Can you work these out from the model? Positions are in its coordinate system, mm. Face numbers are marked on the shaded views. A direction names the side the tool comes from. Round coordinates to 2 decimals unless told otherwise and drop trailing zeros. Order: outer loops, then holes, each group sorted by start corner. A loop starts at its lowest first (then second) coordinate and runs counter-clockwise, first axis right, second up. Notation, with made-up numbers: (-20, -6) -> (7, -6) arc R9 ccw to (7, 4) -> close; hole circle Ø5 at (19.5, -15). An arc over 180 degrees is marked (long way). Use a Markdown table: item, result. Add a question column.
Q1. I'm going to push flat-ended pins straight in: pin 1 Ø2 at (x, z) = (5, 12) entering from +Y; pin 2 Ø3 at (x, z) = (4, 12.5) entering from -Y; pin 3 Ø1.2 at (y, z) = (6, 11) entering from -X. Where does each tip first touch, or does it pass through?
Q2. If we section it at A-A on y = 6: List the corners of the cut face in (x, z) for me, plus the area to 3 significant figures.
Q3. I need wall thicknesses on line 1 along Z through (x, y) = (1, 7); line 2 along X through (y, z) = (5.95, 11). Which ranges of each line are inside material? Lowest first, please. Write a range as [from, to].
Q4. If we section it at D-D on x = 9: List the corners of the cut face in (y, z) for me, plus the area to 3 significant figures.
Q5. If we section it at C-C on z = 12.75: List the corners of the cut face in (x, y) for me.
Q6. For the marked faces 1, 2, 3, 4 and 5, which set-ups out of +Z, -Z, +X, -X, +Y, -Y let a thin tool reach every point of the face, with its end or its side?
Q7. If we section it at B-B on x = 4.25: List the corners of the cut face in (y, z) for me, plus the area to 3 significant figures.
```python
from build123d import *

# Parameters (mm, degrees)
BOX_W              = 10
BOX_H              = 10
BOX_DEPTH          = 10
SKETCH_W           = 4.4
SKETCH_H           = 4.4
PAD_DEPTH          = 4
PAD_FACE4_W        = 10
PAD_FACE4_H        = 10
POCKET_DEPTH       = 2.5
POCKET_FACE5_W     = 10
POCKET_FACE5_H     = 10
POCKET001_DEPTH    = 2.5
SKETCH001_W        = 5
SKETCH001_H        = 10
PAD001_DEPTH       = 10
SKETCH002_W        = 4.4
SKETCH002_H        = 4.4
PAD002_DEPTH       = 4
PAD002_FACE22_W    = 4.4
PAD002_FACE22_H    = 4.4
POCKET002_DEPTH    = 5
POCKET002_FACE16_W = 5
POCKET002_FACE16_H = 10
POCKET003_DEPTH    = 7.5
POCKET003_FACE15_W = 5
POCKET003_FACE15_H = 10
POCKET004_DEPTH    = 2.5
PAD003_DEPTH       = 5


with BuildPart() as part:
    # Box → Box (new body)
    with BuildSketch(Plane.XY):
        with Locations((5, 5)):
            Rectangle(BOX_W, BOX_H)
    extrude(amount=BOX_DEPTH)

    # Sketch (on Face6 of BaseFeature) → Pad (new body)
    with BuildSketch(Plane.XY.offset(10)):
        with Locations((5, 5)):
            Rectangle(SKETCH_W, SKETCH_H)
    extrude(amount=PAD_DEPTH)

    # Pad Face4 → Pocket (cut)
    with BuildSketch(Plane(origin=(5, 10, 5), x_dir=(1, 0, 0), z_dir=(0, 1, 0))):
        Rectangle(PAD_FACE4_W, PAD_FACE4_H)
    extrude(amount=-POCKET_DEPTH, mode=Mode.SUBTRACT)

    # Pocket Face5 → Pocket001 (cut)
    with BuildSketch(Plane(origin=(5, 0, 5), x_dir=(-1, 0, 0), z_dir=(0, -1, 0))):
        Rectangle(POCKET_FACE5_W, POCKET_FACE5_H)
    extrude(amount=-POCKET001_DEPTH, mode=Mode.SUBTRACT)

    # Sketch001 (on Face3 of Pocket001) → Pad001 (join)
    with BuildSketch(Plane(origin=(0, 7.5, 0), x_dir=(-1, 0, 0), z_dir=(0, 1, 0))):
        with Locations((-5, 5)):
            Rectangle(SKETCH001_W, SKETCH001_H)
    extrude(amount=PAD001_DEPTH)

    # Sketch002 (on Face6 of Pad001) → Pad002 (join)
    with BuildSketch(Plane.XY.offset(10)):
        with Locations((5, 12.5)):
            Rectangle(SKETCH002_W, SKETCH002_H)
    extrude(amount=PAD002_DEPTH)

    # Pad002 Face22 → Pocket002 (cut)
    with BuildSketch(Plane(origin=(5, 12.5, 14), x_dir=(0, 1, 0), z_dir=(0, 0, 1))):
        Rectangle(PAD002_FACE22_W, PAD002_FACE22_H)
    extrude(amount=-POCKET002_DEPTH, mode=Mode.SUBTRACT)

    # Pocket002 Face16 → Pocket003 (cut)
    with BuildSketch(Plane(origin=(5, 17.5, 5), x_dir=(1, 0, 0), z_dir=(0, 1, 0))):
        Rectangle(POCKET002_FACE16_W, POCKET002_FACE16_H)
    extrude(amount=-POCKET003_DEPTH, mode=Mode.SUBTRACT)

    # Pocket003 Face15 → Pocket004 (cut)
    with BuildSketch(Plane(origin=(5, 10, 5), x_dir=(1, 0, 0), z_dir=(0, 1, 0))):
        Rectangle(POCKET003_FACE15_W, POCKET003_FACE15_H)
    extrude(amount=-POCKET004_DEPTH, mode=Mode.SUBTRACT)

    # Pocket004 Face4 → Pad003 (add)
    with BuildSketch(Plane(origin=(5, 5, 0), x_dir=(0, -1, 0), z_dir=(0, 0, -1))):
        Polygon((2.5, 5), (-2.5, 5), (-2.5, 2.5), (-2.5, -2.5), (-2.5, -5), (2.5, -5), align=None)
    extrude(amount=PAD003_DEPTH)


solid = part.part
```
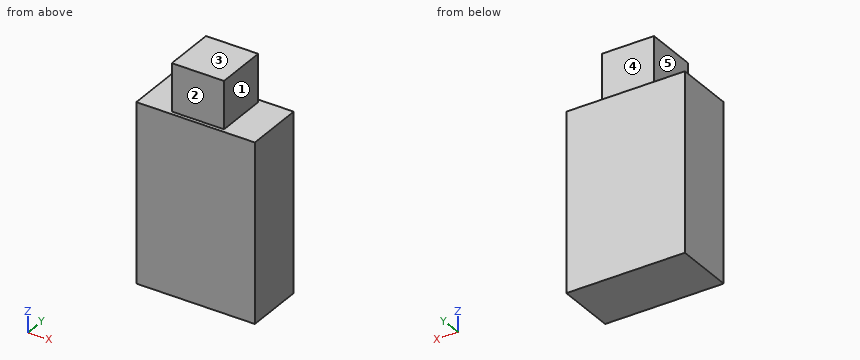
Answer below:
| question | item | result |
|---|---|---|
| 1 | pin 1 | y = 7.2 |
| 1 | pin 2 | y = 2.8 |
| 1 | pin 3 | x = 2.8 |
| 2 | outline | (0, -5) -> (10, -5) -> (10, 10) -> (7.2, 10) -> (7.2, 14) -> (2.8, 14) -> (2.8, 10) -> (0, 10) -> close |
| 2 | area | 168 mm² |
| 3 | line 1 | [-5, 10] |
| 3 | line 2 | [2.8, 7.2] |
| 4 | outline | (2.5, -5) -> (7.5, -5) -> (7.5, 10) -> (2.5, 10) -> close |
| 4 | area | 75.0 mm² |
| 5 | outline | (2.8, 2.8) -> (7.2, 2.8) -> (7.2, 7.2) -> (2.8, 7.2) -> close |
| 6 | face 1 | +Z, +X, +Y, -Y |
| 6 | face 2 | +Z, +X, -X, -Y |
| 6 | face 3 | +Z, +X, -X, +Y, -Y |
| 6 | face 4 | +Z, +X, -X, +Y |
| 6 | face 5 | +Z, -X, +Y, -Y |
| 7 | outline | (2.5, -5) -> (7.5, -5) -> (7.5, 10) -> (7.2, 10) -> (7.2, 14) -> (2.8, 14) -> (2.8, 10) -> (2.5, 10) -> close |
| 7 | area | 92.6 mm² |
